Read the model definition and answer for the solid it produces. Units are mm, in the model's axes. Give positions to 0.01 mm unless a question says otherwise; leave off trailing zeros. Write each loop counter-clockwise with the first axis right and the second up, starting at its lowest first coordinate (ties: lowest second). Pieces come first, ordered by that corner, then holes. Notation, with made-up numbers: M 17,9.5 L 54,9.5 A27 ccw 54,47.5 Z; hole C 15.25,-25.5 d10. An arc over 180 degrees is marked long. Use a Markdown table: item, result. Add a question column.
Item 1: A cutting plane is placed at A-A on z = -6.35. Determine the outline of the cut face in (x, y), then the cut area to 3 significant figures.
Item 2: The mould has two halves that part along Z. Classify faces 1 (the cylindrical face through (12.522, 13.389, -41.517)), 2 (the flat face through (0, 11, -6)), 3 (the cylindrical face through (12.697, 14.809, -25.121)), 4 (the flat face through (13, 14, -50.8)): pulls with the +Z half, pulls with the -Z half, needs draft (parallel to the pull), parting line crosses it, or undercut.
Item 3: A cutting plane is placed at C-C on y = 10.5. Determine the outline of the cut face in (x, z), then the cut area to 3 significant figures.
Item 4: A cutting plane is placed at D-D on x = 21.5. Determine the outline of the cut face in (y, z) (3 decimals), then the cut area to 3 significant figures.
Item 5: Given P1, Ø1, axis at x = 22, z = -38.5, coming from the -Y side; P2, Ø1.5, axis at y = 8.5, z = -32, coming from the -X side; P3, Ø4, axis at y = 14.605, z = -6.35, coming from the -X side, each flat-ended and moving along its own axis, determine where each tip first touches the part or whether it passes through.
Item 6: A cutting plane is placed at B-B on x = 4.5. Determine the outline of the cut face in (y, z) (3 decimals).
Item 7: Consider probe 1 along Z at (x, y) = (19, 14.5); probe 2 along Y at (x, z) = (13.25, -6.5); probe 3 along Z at (x, y) = (21.25, 13.5). Determine where each line is inside the solid, lowest interval first. Write a range as [from, to].
from build123d import *

# Parameters (mm, degrees)
SKETCH1_W           = 25.4
SKETCH1_H           = 50.8
BOSS_EXTRUDE1_DEPTH = 29.21
SKETCH2_R           = 12.7
CUT_EXTRUDE1_DEPTH  = 64.86723808
SKETCH4_R           = 3.175
CUT_EXTRUDE2_DEPTH  = 64.86723808
SKETCH5_R           = 3.175
CUT_EXTRUDE3_DEPTH  = 64.86723808


with BuildPart() as part:
    # Sketch1 → Boss-Extrude1 (new body)
    with BuildSketch(Plane(origin=(0, 0, 0), x_dir=(1, 0, 0), z_dir=(0, 1, 0))):
        with Locations((12.7, 25.4)):
            Rectangle(SKETCH1_W, SKETCH1_H)
    extrude(amount=BOSS_EXTRUDE1_DEPTH)

    # Sketch2 → Cut-Extrude1 (cut, through all)
    with BuildSketch(Plane(origin=(0, 29.21, 0), x_dir=(1, 0, 0), z_dir=(0, 1, 0))):
        with Locations((0, 25.4)):
            Circle(SKETCH2_R)
    extrude(amount=-CUT_EXTRUDE1_DEPTH, mode=Mode.SUBTRACT)

    # Sketch4 → Cut-Extrude2 (cut, through all)
    with BuildSketch(Plane.ZY):
        with Locations((-44.45, 14.605)):
            Circle(SKETCH4_R)
    extrude(amount=-CUT_EXTRUDE2_DEPTH, mode=Mode.SUBTRACT)

    # Sketch5 → Cut-Extrude3 (cut, through all)
    with BuildSketch(Plane.ZY):
        with Locations((-6.35, 14.605)):
            Circle(SKETCH5_R)
    extrude(amount=-CUT_EXTRUDE3_DEPTH, mode=Mode.SUBTRACT)


solid = part.part
Filled in:
| question | item | result |
|---|---|---|
| 1 | outline | M 0,0 L 25.4,0 L 25.4,11.43 L 0,11.43 Z; M 0,17.78 L 25.4,17.78 L 25.4,29.21 L 0,29.21 Z |
| 1 | area | 581 mm² |
| 2 | face 1 | undercut |
| 2 | face 2 | needs draft |
| 2 | face 3 | undercut |
| 2 | face 4 | pulls with the -Z half |
| 3 | outline | M 0,-50.8 L 25.4,-50.8 L 25.4,0 L 0,0 L 0,-12.7 A12.7 cw 0,-38.1 Z |
| 3 | area | 1,040 mm² |
| 4 | outline | M 0,-50.8 L 29.21,-50.8 L 29.21,0 L 0,0 Z; hole C 14.605,-44.45 d6.35; hole C 14.605,-6.35 d6.35 |
| 4 | area | 1,420 mm² |
| 5 | P1 | y = 0 |
| 5 | P2 | x = 10.36 |
| 5 | P3 | through |
| 6 | outline | M 0,-50.8 L 29.21,-50.8 L 29.21,-37.276 L 0,-37.276 Z; M 0,-13.524 L 29.21,-13.524 L 29.21,0 L 0,0 Z; hole C 14.605,-44.45 d6.35; hole C 14.605,-6.35 d6.35 |
| 7 | probe 1 | [-50.8, -47.62], [-41.28, -9.52], [-3.18, 0] |
| 7 | probe 2 | [0, 11.43], [17.78, 29.21] |
| 7 | probe 3 | [-50.8, -47.43], [-41.47, -9.33], [-3.37, 0] |
